Input: part model. Units: mm. Frame: model coordinates. A direction names the side the tool comes from. Give positions to 0.01 mm unless a question says otherwise; leave off trailing zeros. Order: outer loops, then holes, each group sorted by start corner. A loop starts at its lowest first (then second) coordinate and runs counter-clockwise, first axis right, second up. Notation, with made-up numbers: (-27, 67) - (-14, 67) arc R18 ccw to (-14, 77) - close; hole circle Ø9 at (24.5, 18.25). An arc over 180 degrees is marked (long way). Use a Markdown table: item, result.
Autodesk Inventor part; units mm, degrees
ref_plane "YZ Plane" through (0, 0, 0) normal (1, 0, 0) x (0, 1, 0)
ref_plane "XZ Plane" through (0, 0, 0) normal (0, 1, 0) x (-1, 0, 0)
ref_plane "XY Plane" through (0, 0, 0) normal (0, 0, 1) x (1, 0, 0)
sketch "Skizze1" plane through (0, 0, 0) normal (0, 1, 0) x (-1, 0, 0)
  line L0 (4.3, 1.85) -> (-4.3, 1.85)
  line L1 (-4.3, 1.85) -> (-4.3, -1.85)
  line L2 (-4.3, -1.85) -> (4.3, -1.85)
  line L3 (4.3, -1.85) -> (4.3, 1.85)
  line L4 (4.3, 1.85) -> (-4.3, -1.85) construction
  line L5 (-4.3, 1.85) -> (4.3, -1.85) construction
  point P0 (0, 0)
  dimension "d0" = 8.6
  dimension "d1" = 3.7
extrude "Extrusion1" add sketch "Skizze1" along normal blind 3.5
sketch "Skizze2" plane through (0, 3.5, 0) normal (0, 1, 0) x (1, 0, 0)
  line L0 (-1.75, -0.7) -> (1.75, -0.7)
  line L1 (1.75, -0.7) -> (1.75, 0.7)
  line L2 (1.75, 0.7) -> (-1.75, 0.7)
  line L3 (-1.75, 0.7) -> (-1.75, -0.7)
  line L4 (-1.75, -0.7) -> (1.75, 0.7) construction
  line L5 (1.75, -0.7) -> (-1.75, 0.7) construction
  line L6 (-1.95, -0.9) -> (1.95, -0.9)
  line L7 (1.95, -0.9) -> (1.95, 0.9)
  line L8 (1.95, 0.9) -> (-1.95, 0.9)
  line L9 (-1.95, 0.9) -> (-1.95, -0.9)
  line L10 (-1.95, -0.9) -> (1.95, 0.9) construction
  line L11 (1.95, -0.9) -> (-1.95, 0.9) construction
  point P0 (0, 0)
  dimension "d4" = 1.4
  dimension "d5" = 3.5
  dimension "d6" = 0.2
  dimension "d7" = 0.2
extrude "Extrusion2" cut sketch "Skizze2" against normal blind 0.1
sketch "Skizze3" plane through (0, 3.5, 0) normal (0, 1, 0) x (1, 0, 0)
  line L0 (-1.75, 0.7) -> (-1.75, -0.7)
  line L1 (1.75, 0.7) -> (-1.75, 0.7)
  line L2 (-1.75, -0.7) -> (1.75, -0.7)
  line L3 (-1.75, 0.7) -> (-0.35, 0.7)
  line L4 (-0.35, 0.7) -> (-0.35, -0.7)
  line L5 (-0.35, -0.7) -> (-1.75, -0.7)
  line L6 (-1.75, -0.7) -> (-1.75, 0.7)
  point P0 (0, 0)
  dimension "d10" = 1.4
extrude "Extrusion3" add sketch "Skizze3" along normal blind 2.8
sketch "Skizze4" plane through (0, 0, 0) normal (0, -1, 0) x (1, 0, 0)
  circle A0 centre (-0.2, 0) radius 1
  circle A1 centre (2.8, 0) radius 1
  line L0 (4.3, 1.85) -> (4.3, -1.85)
  point P0 (0, 0)
  dimension "d16" = 1.5
  dimension "d17" = 3
  dimension "d18" = 2
extrude "Extrusion4" add sketch "Skizze4" along normal blind 5
fillet "Rundung1" radius 0.2 20 edges at (0, 3.5, 1.85) (4.3, 3.5, 0) (4.3, 1.75, 1.85) (4.3, 0, 0) (4.3, 1.75, -1.85) (0, 3.5, -1.85) (0, 0, -1.85) (-4.3, 1.75, -1.85) (-4.3, 0, 0) (-4.3, 1.75, 1.85) (-4.3, 3.5, 0) (0, 0, 1.85) (-0.35, 4.9, -0.7) (-1.75, 4.85, -0.7) (-1.75, 4.85, 0.7) (-0.35, 4.9, 0.7) (-1.05, 6.3, 0.7) (-0.35, 6.3, 0) (-1.05, 6.3, -0.7) (-1.75, 6.3, 0)
chamfer "Fasen1" distance 0.2 angle 45 2 edges at (-1.2, 0, 0) (1.8, 0, 0)
properties part number "Schalter"
1. Set-up query: faces 1 (the face through (-0.35, 5, 0)), 2 (the face through (-1, 5, -0.7)), 3 (the face through (3.724, -2.566, 0.383)). Return all of +Z, -Z, +X, -X, +Y, -Y with unobstructed straight access to the full face (end or side cutting, diameter ignored); none if empty.
Response:
| item | result |
|---|---|
| face 1 | +Z, -Z, +X, +Y |
| face 2 | +Y |
| face 3 | -Y |
2. Section query B-B (x = -0.2). Return loops of the section in (y, z).
Response:
| item | result |
|---|---|
| outline | (-5, -1) - (-0.2, -1) - (0, -1.2) - (0, -1.65) arc R0.2 ccw to (0.2, -1.85) - (3.3, -1.85) arc R0.2 ccw to (3.5, -1.65) - (3.5, -0.9) - (3.4, -0.9) - (3.4, -0.7) - (3.5, -0.7) - (3.5, 0.7) - (3.4, 0.7) - (3.4, 0.9) - (3.5, 0.9) - (3.5, 1.65) arc R0.2 ccw to (3.3, 1.85) - (0.2, 1.85) arc R0.2 ccw to (0, 1.65) - (0, 1.2) - (-0.2, 1) - (-5, 1) - close |
3. Pin query (flat end, axial travel): pin 1 (1.1 mm diameter, centred on x = 1, z = 0, fed in from +Y); pin 2 (0.8 mm diameter, centred on y = 5, z = 0, fed in from +X); pin 3 (0.8 mm diameter, centred on y = 4, z = 0, fed in from -X). Return the tip coordinate at first contact, or that it passes through.
Response:
| item | result |
|---|---|
| pin 1 | stops at y = 3.5 |
| pin 2 | stops at x = -0.35 |
| pin 3 | stops at x = -1.75 |
4. Section query A-A (y = 3.75). Return loops of the section in (x, z), then the cut area to 3 significant figures.
Response:
| item | result |
|---|---|
| outline | (-1.75, -0.5) arc R0.2 ccw to (-1.55, -0.7) - (-0.55, -0.7) arc R0.2 ccw to (-0.35, -0.5) - (-0.35, 0.5) arc R0.2 ccw to (-0.55, 0.7) - (-1.55, 0.7) arc R0.2 ccw to (-1.75, 0.5) - close |
| area | 1.93 mm^2 |
5. Section query D-D (y = -3). Return loops of the section in (x, z), then the cut area to 3 significant figures.
Response:
| item | result |
|---|---|
| outline | circle Ø2 at (-0.2, 0); circle Ø2 at (2.8, 0) |
| area | 6.28 mm^2 |
6. Material intervals for line 1 along X through (y, z) = (-0.25, -0.05); line 2 along Y through (x, z) = (-2.5, 0.9); line 3 along X through (y, z) = (-2.25, -0.4), sorted ascending.
Response:
| item | result |
|---|---|
| line 1 | x = -1.2 to 0.8, 1.8 to 3.8 |
| line 2 | y = 0 to 3.5 |
| line 3 | x = -1.12 to 0.72, 1.88 to 3.72 |
7. Mould query, pull axis X, two halves, no side actions, for faces 4 (the face through (4.3, 2, 0)), 5 (the face through (-4.3, 2, 0)), 6 (the face through (0.1, 3.5, 1.1)), 7 (the face through (-2, 0, 0)). Classes: pulls with the +X half, pulls with the -X half, needs draft (parallel to the pull), parting line crosses it, or undercut.
Response:
| item | result |
|---|---|
| face 4 | pulls with the +X half |
| face 5 | pulls with the -X half |
| face 6 | needs draft |
| face 7 | undercut |
